Model file for the job. Use its own axes, mm. A direction names the side the tool comes from. Round coordinates to 2 decimals unless told otherwise and drop trailing zeros. Loops run counter-clockwise (first coordinate to the right, second up) from the corner with the lowest first, then second, coordinate; pieces in that order, holes last. Notation, with made-up numbers: M 27,41 L 71,41 A21 cw 71,61 Z; hole C 81,-3.75 d9. An arc over 180 degrees is marked long. Use a Markdown table: item, result. Add a question column.
Q1. Cut at A-A (y = 40.5). Give the cut face in (x, z), plus the area to 3 significant figures.
Q2. Cut at C-C (z = 23). Give the cut face in (x, y).
Q3. Mould opens along X. For faces 1 (the face through (5.135, 28, 9)), 2 (the face through (-53.45, 19.52, 28.04)), 3 (the face through (-11, 28, 38.862)), 4 (the face through (-13.734, 14.438, 28.045)) say: +X half, -X half, draft (parallel to the pull), parting line (faces both ways), or undercut.
Q4. Probe line 1 (Z direction, x = -25.5, y = 17); line 2 (X direction, y = 31, z = 30); line 3 (X direction, y = 21.5, z = 21). List the from-to ranges inside material, lowest first. Write a range as from..to.
Q5. Cut at D-D (x = -39). Give the cut face in (y, z).
Q6. Cut at B-B (x = -31). Give the cut face in (y, z), plus the area to 3 significant figures.
Q7. Tool access for faces 5 (the face through (-27, 28, 17.526)), 6 (the face through (-27, 28, 0)): list every direction of +Z, -Z, +X, -X, +Y, -Y with a clear straight run to the whole face (end or side of a thin tool).
Q8. Pin check, flat tips, straight feed: pin 1 (12 mm diameter, centred on x = -46.5, z = 29, fed in from -Y); pin 2 (2 mm diameter, centred on x = -27.5, y = 39, fed in from +Z); pin 3 (3 mm diameter, centred on y = 24, z = 28.5, fed in from +X). Stop position of each tip, or through.
from build123d import *

# Parameters (mm, degrees)
F1_DEPTH = 17.526
F2_R     = 13.808948
F3_DEPTH = 21.336


with BuildPart() as f1:
    # F0 (on Top) → F1 (new body)
    with BuildSketch(Plane.XY):
        Polygon((-50.618237, 43.793876), (-58.365237, 43.793876), (-58.365237, 36.300876), (-57.095237, 36.300876), (-57.095237, 36.173876), (-57.095237, 36.046876), (-58.365237, 36.046876), (-58.365237, 20.044876), (-57.095237, 20.044876), (-57.095237, 19.917876), (-57.095237, 19.790876), (-58.365237, 19.790876), (-58.365237, 12.043876), (-50.618237, 12.043876), (-50.618237, 18.393876), (-50.491237, 18.393876), (-50.364237, 18.393876), (-50.364237, 12.043876), (-33.346237, 12.043876), (-33.346237, 18.393876), (-33.219237, 18.393876), (-33.092237, 18.393876), (-33.092237, 12.043876), (-26.615237, 12.043876), (-26.615237, 19.790876), (-27.885237, 19.790876), (-27.885237, 19.917876), (-27.885237, 20.044876), (-26.615237, 20.044876), (-26.615237, 36.046876), (-27.885237, 36.046876), (-27.885237, 36.173876), (-27.885237, 36.300876), (-26.615237, 36.300876), (-26.615237, 43.793876), (-33.092237, 43.793876), (-33.092237, 37.443876), (-33.219237, 37.443876), (-33.346237, 37.443876), (-33.346237, 43.793876), (-50.364237, 43.793876), (-50.364237, 37.443876), (-50.491237, 37.443876), (-50.618237, 37.443876), align=None)
        Polygon((-50.364237, 43.793876), (-50.618237, 43.793876), (-50.618237, 37.443876), (-50.491237, 37.443876), (-50.364237, 37.443876), align=None)
        Polygon((-57.095237, 36.300876), (-58.365237, 36.300876), (-58.365237, 36.173876), (-58.365237, 36.046876), (-57.095237, 36.046876), (-57.095237, 36.173876), align=None)
        Polygon((-33.092237, 43.793876), (-33.346237, 43.793876), (-33.346237, 37.443876), (-33.219237, 37.443876), (-33.092237, 37.443876), align=None)
        Polygon((-57.095237, 20.044876), (-58.365237, 20.044876), (-58.365237, 19.917876), (-58.365237, 19.790876), (-57.095237, 19.790876), (-57.095237, 19.917876), align=None)
        Polygon((-20.138237, 43.793876), (-26.615237, 43.793876), (-26.615237, 36.300876), (-25.345237, 36.300876), (-25.345237, 36.173876), (-25.345237, 36.046876), (-26.615237, 36.046876), (-26.615237, 20.044876), (-25.345237, 20.044876), (-25.345237, 19.917876), (-25.345237, 19.790876), (-26.615237, 19.790876), (-26.615237, 12.043876), (-20.138237, 12.043876), (-20.138237, 18.393876), (-20.011237, 18.393876), (-19.884237, 18.393876), (-19.884237, 12.043876), (-2.866237, 12.043876), (-2.866237, 18.393876), (-2.739237, 18.393876), (-2.612237, 18.393876), (-2.612237, 12.043876), (5.134763, 12.043876), (5.134763, 19.790876), (3.864763, 19.790876), (3.864763, 19.917876), (3.864763, 20.044876), (5.134763, 20.044876), (5.134763, 36.046876), (3.864763, 36.046876), (3.864763, 36.173876), (3.864763, 36.300876), (5.134763, 36.300876), (5.134763, 43.793876), (-2.612237, 43.793876), (-2.612237, 37.443876), (-2.739237, 37.443876), (-2.866237, 37.443876), (-2.866237, 43.793876), (-19.884237, 43.793876), (-19.884237, 37.443876), (-20.011237, 37.443876), (-20.138237, 37.443876), align=None)
        Polygon((-19.884237, 43.793876), (-20.138237, 43.793876), (-20.138237, 37.443876), (-20.011237, 37.443876), (-19.884237, 37.443876), align=None)
        Polygon((-2.612237, 43.793876), (-2.866237, 43.793876), (-2.866237, 37.443876), (-2.739237, 37.443876), (-2.612237, 37.443876), align=None)
        Polygon((-50.618237, 18.393876), (-50.618237, 12.043876), (-50.491237, 12.043876), (-50.364237, 12.043876), (-50.364237, 18.393876), (-50.491237, 18.393876), align=None)
        Polygon((5.134763, 36.046876), (5.134763, 36.300876), (3.864763, 36.300876), (3.864763, 36.173876), (3.864763, 36.046876), align=None)
        Polygon((-33.219237, 12.043876), (-33.092237, 12.043876), (-33.092237, 18.393876), (-33.219237, 18.393876), (-33.346237, 18.393876), (-33.346237, 12.043876), align=None)
        Polygon((-20.138237, 18.393876), (-20.138237, 12.043876), (-19.884237, 12.043876), (-19.884237, 18.393876), (-20.011237, 18.393876), align=None)
        Polygon((5.134763, 19.790876), (5.134763, 20.044876), (3.864763, 20.044876), (3.864763, 19.917876), (3.864763, 19.790876), align=None)
        Polygon((-2.866237, 18.393876), (-2.866237, 12.043876), (-2.612237, 12.043876), (-2.612237, 18.393876), (-2.739237, 18.393876), align=None)
        Polygon((-26.615237, 36.046876), (-26.615237, 36.300876), (-27.885237, 36.300876), (-27.885237, 36.173876), (-27.885237, 36.046876), align=None)
        Polygon((-25.345237, 36.300876), (-26.615237, 36.300876), (-26.615237, 36.046876), (-25.345237, 36.046876), (-25.345237, 36.173876), align=None)
        Polygon((-25.345237, 20.044876), (-26.615237, 20.044876), (-26.615237, 19.790876), (-25.345237, 19.790876), (-25.345237, 19.917876), align=None)
        Polygon((-26.615237, 19.790876), (-26.615237, 20.044876), (-27.885237, 20.044876), (-27.885237, 19.917876), (-27.885237, 19.790876), align=None)
    extrude(amount=F1_DEPTH)

    # F2 (on face) → F3 (join)
    with BuildSketch(Plane.XY.offset(17.526)):
        with Locations((-42.490237, 27.918876)):
            Circle(F2_R)
        with Locations((-10.740237, 27.918876)):
            Circle(F2_R)
    extrude(amount=F3_DEPTH)


solid = f1.part
Checked values:
| question | item | result |
|---|---|---|
| 1 | outline | M -58.37,0 L 5.13,0 L 5.13,17.53 L -5.05,17.53 L -5.05,38.86 L -16.43,38.86 L -16.43,17.53 L -36.8,17.53 L -36.8,38.86 L -48.18,38.86 L -48.18,17.53 L -58.37,17.53 Z |
| 1 | area | 1,600 mm^2 |
| 2 | outline | C -42.49,27.92 d27.62; C -10.74,27.92 d27.62 |
| 3 | face 1 | +X half |
| 3 | face 2 | undercut |
| 3 | face 3 | draft |
| 3 | face 4 | undercut |
| 4 | line 1 | z = 0..17.53 |
| 4 | line 2 | x = -55.95..-29.03, -24.2..2.72 |
| 4 | line 3 | x = -54.72..-30.26, -22.97..1.49 |
| 5 | outline | M 12.04,0 L 43.79,0 L 43.79,17.53 L 41.28,17.53 L 41.28,38.86 L 14.56,38.86 L 14.56,17.53 L 12.04,17.53 Z |
| 6 | outline | M 12.04,0 L 43.79,0 L 43.79,17.53 L 35.58,17.53 L 35.58,38.86 L 20.26,38.86 L 20.26,17.53 L 12.04,17.53 Z |
| 6 | area | 883 mm^2 |
| 7 | face 5 | +Z |
| 7 | face 6 | -Z, +X, -X, +Y, -Y |
| 8 | pin 1 | stops at y = 14.11 |
| 8 | pin 2 | stops at z = 17.53 |
| 8 | pin 3 | stops at x = 2.86 |
